from build123d import *

# Parameters (mm, degrees)
F1_DEPTH = 45.72
F0_R     = 14.2875
F2_DEPTH = 25.908


with BuildPart() as f1:
    # F0 (on Front) → F1 (new body)
    with BuildSketch(Plane.XZ):
        with BuildLine():
            Line((9.5121844836, 26.9452959039), (0, 28.575))
            ThreePointArc((0, 28.575), (-28.575, 0), (0, -28.575))
            Line((0, -28.575), (9.5121844836, -26.9452959039))
            ThreePointArc((9.5121844836, -26.9452959039), (23.3274655355, -16.5033322905), (28.575, 0))
            ThreePointArc((28.575, 0), (23.3274655355, 16.5033322905), (9.5121844836, 26.9452959039))
        make_face()
        with BuildLine():
            ThreePointArc((-13.4703841816, 4.7625), (0, 14.2875), (13.4703841816, 4.7625))
            Line((13.4703841816, 4.7625), (21.229936273, 4.7625))
            Line((21.229936273, 4.7625), (21.229936273, -4.7625))
            Line((21.229936273, -4.7625), (13.4703841816, -4.7625))
            ThreePointArc((13.4703841816, -4.7625), (0, -14.2875), (-13.4703841816, -4.7625))
            Line((-13.4703841816, -4.7625), (-16.870063727, -4.7625))
            Line((-16.870063727, -4.7625), (-16.870063727, 4.7625))
            Line((-16.870063727, 4.7625), (-13.4703841816, 4.7625))
        make_face(mode=Mode.SUBTRACT)
        with BuildLine():
            ThreePointArc((-13.4703841816, -4.7625), (-14.2875, 0), (-13.4703841816, 4.7625))
            Line((-13.4703841816, 4.7625), (-16.870063727, 4.7625))
            Line((-16.870063727, 4.7625), (-16.870063727, -4.7625))
            Line((-16.870063727, -4.7625), (-13.4703841816, -4.7625))
        make_face()
    extrude(amount=F1_DEPTH)

    # F0 (on Front) → F2 (join)
    with BuildSketch(Plane.XZ):
        with BuildLine():
            Line((9.5121844836, 26.9452959039), (0, 28.575))
            ThreePointArc((0, 28.575), (-28.575, 0), (0, -28.575))
            Line((0, -28.575), (9.5121844836, -26.9452959039))
            ThreePointArc((9.5121844836, -26.9452959039), (23.3274655355, -16.5033322905), (28.575, 0))
            ThreePointArc((28.575, 0), (23.3274655355, 16.5033322905), (9.5121844836, 26.9452959039))
        make_face()
        with BuildLine():
            ThreePointArc((-13.4703841816, 4.7625), (0, 14.2875), (13.4703841816, 4.7625))
            Line((13.4703841816, 4.7625), (21.229936273, 4.7625))
            Line((21.229936273, 4.7625), (21.229936273, -4.7625))
            Line((21.229936273, -4.7625), (13.4703841816, -4.7625))
            ThreePointArc((13.4703841816, -4.7625), (0, -14.2875), (-13.4703841816, -4.7625))
            Line((-13.4703841816, -4.7625), (-16.870063727, -4.7625))
            Line((-16.870063727, -4.7625), (-16.870063727, 4.7625))
            Line((-16.870063727, 4.7625), (-13.4703841816, 4.7625))
        make_face(mode=Mode.SUBTRACT)
        with BuildLine():
            ThreePointArc((9.5121844836, 26.9452959039), (4.8253908933, 28.1646272428), (0, 28.575))
            Line((0, 28.575), (9.5121844836, 26.9452959039))
        make_face()
        with BuildLine():
            Line((9.5121844836, -26.9452959039), (0, -28.575))
            ThreePointArc((0, -28.575), (4.8253908933, -28.1646272428), (9.5121844836, -26.9452959039))
        make_face()
        with BuildLine():
            Line((57.1919272622, 18.7764181619), (9.5121844836, 26.9452959039))
            ThreePointArc((9.5121844836, 26.9452959039), (23.3274655355, 16.5033322905), (28.575, 0))
            ThreePointArc((28.575, 0), (23.3274655355, -16.5033322905), (9.5121844836, -26.9452959039))
            Line((9.5121844836, -26.9452959039), (57.1919272622, -18.7764181619))
            ThreePointArc((57.1919272622, -18.7764181619), (34.925, 0), (57.1919272622, 18.7764181619))
        make_face()
        with BuildLine():
            ThreePointArc((73.025, 0), (68.5383952831, 12.2804730295), (57.1919272622, 18.7764181619))
            ThreePointArc((57.1919272622, 18.7764181619), (34.925, 0), (57.1919272622, -18.7764181619))
            ThreePointArc((57.1919272622, -18.7764181619), (68.5383952831, -12.2804730295), (73.025, 0))
        make_face()
        with Locations((53.975, 0)):
            Circle(F0_R, mode=Mode.SUBTRACT)
    extrude(amount=F2_DEPTH)


solid = f1.part
Design review of the part built by this model. Coordinates are the model's own, in mm. A direction names the side the tool comes from. Round coordinates to 2 decimals unless told otherwise and drop trailing zeros. Loops run counter-clockwise (first coordinate to the right, second up) from the corner with the lowest first, then second, coordinate; pieces in that order, holes last. Notation, with made-up numbers: M 81.25,54.25 L 88.25,54.25 A7 cw 88.25,60.25 Z; hole C 44,-7 d7. An arc over 180 degrees is marked long. Answer as a JSON object with one key per item and string values.
Item 1: Clearance check with flat-ended pins moving along their axes: P1, Ø1.5, axis at x = 14, y = -17.5, coming from the +Z side; P2, Ø0.5, axis at x = 5.5, z = -28, coming from the -Y side; P3, Ø2.5, axis at x = 16.5, y = -27, coming from the +Z side; P4, Ø6, axis at x = 10, z = 2.5, coming from the -Y side. State where each tip first meets the part, or that it passes through.
Answer sheet:
{"P1": "stops at z = 26.3", "P2": "stops at y = -25.91", "P3": "stops at z = 25.85", "P4": "passes through"}
Item 2: Machinability: for faces 1 (the flat face through (22, 0, 0)), 2 (the flat face through (4.69, -35.68, -27.77)), 3 (the flat face through (-13, -45.72, 7)), 4 (the flat face through (17, -23, -4.762)), 5 (the flat face through (4.82, -35.68, 27.75)), which of the approach directions +Z, -Z, +X, -X, +Y, -Y give a long, thin tool a straight path to every point of the face, cutting with its end or side? Answer none if there is none.
Answer sheet:
{"face 1": "+Z, -Z, +X, -X, +Y", "face 2": "-Z, +X, -Y", "face 3": "+Z, -Z, +X, -X, -Y", "face 4": "+Y, -Y", "face 5": "+Z, +X, -Y"}
Item 3: We need section B-B on x = 53. Give the boundary of the cut face in (y, z).
Answer sheet:
{"outline": "M -25.91,-19.49 L 0,-19.49 L 0,-14.25 L -25.91,-14.25 Z; M -25.91,14.25 L 0,14.25 L 0,19.49 L -25.91,19.49 Z"}
Item 4: We need section A-A on y = -3.5. State how many separate pieces and enclosed holes the cut face has, and give its area (3 significant figures).
Answer sheet:
{"separate pieces": "1", "enclosed holes": "2", "area": "3,090 mm^2"}
Item 5: The part is to be moulded in two halves that separate along Z. For faces 6 (the flat face through (17, -23, 4.762)), 7 (the flat face through (21.23, -23, 0)), 8 (the flat face through (33.018, -12.773, -22.918)), 9 (the flat face through (39, -25.908, 0)), say which applies: pulls with the +Z half, pulls with the -Z half, needs draft (parallel to the pull), parting line crosses it, or undercut.
Answer sheet:
{"face 6": "undercut", "face 7": "undercut", "face 8": "pulls with the -Z half", "face 9": "needs draft"}
Item 6: Wall thickness on L1, parallel to X at y = -7, z = 0.5; L2, parallel to Y at x = 31.5, z = 12; L3, parallel to X at y = -34.5, z = 3: over which ranges is each line inside the solid? List them lowest first. Write a range as from..to.
Answer sheet:
{"L1": "x = -28.57..-14.28, 21.23..39.7, 68.25..73.02", "L2": "y = -25.91..0", "L3": "x = -28.42..-13.97, 21.23..28.42"}
Item 7: We need section C-C on z = -6. Give the boundary of the cut face in (x, y).
Answer sheet:
{"outline": "M -27.94,-45.72 L -12.97,-45.72 L -12.97,0 L -27.94,0 Z; M 12.97,-45.72 L 27.94,-45.72 L 27.94,-25.91 L 41.01,-25.91 L 41.01,0 L 12.97,0 Z; M 66.94,-25.91 L 72.06,-25.91 L 72.06,0 L 66.94,0 Z"}
